Could you check a few things on this model? Use its own coordinates, in mm. Round coordinates to 2 decimals unless told otherwise and drop trailing zeros. Write each loop counter-clockwise with the first axis right and the second up, starting at its lowest first coordinate (ties: lowest second). Pieces come first, ordered by that corner, then holes. Notation, with made-up numbers: (49, 52) - (73, 52) arc R7 cw to (73, 63) - close; hole circle Ø7 at (-10, 29). An arc over 180 degrees is marked (long way). Put each result on its own line as item: value.
from build123d import *

# Parameters (mm, degrees)
SKETCH1_W                   = 50.8
SKETCH1_H                   = 88.500000038
SKETCH1_R                   = 14.2621
BOSS_EXTRUDE1_DEPTH         = 3.175
FILLET1_R                   = 5.08
F_1_4_0_25_DIAMETER_HOLE2_D = 6.35


with BuildPart() as part:
    # Sketch1 → Boss-Extrude1 (new, symmetric)
    with BuildSketch(Plane(origin=(0, 0, 0), x_dir=(0, 0, -1), z_dir=(1, 0, 0))):
        Rectangle(SKETCH1_W, SKETCH1_H)
        with Locations((0, -12.500000019)):
            Circle(SKETCH1_R, mode=Mode.SUBTRACT)
    extrude(amount=BOSS_EXTRUDE1_DEPTH, both=True)

    # Fillet1
    fillet1_edges = [part.edges().sort_by_distance(p)[0] for p in [
        (0, -44.250000019, -25.4),
        (0, -44.250000019, 25.4),
        (0, 44.250000019, 25.4),
        (0, 44.250000019, -25.4),
    ]]
    fillet(fillet1_edges, radius=FILLET1_R)

    # 1/4 (0.25) Diameter Hole2 (through all)
    with Locations(Plane(origin=(3.175, -37.900000019, 19.05), x_dir=(0, 0, 1), z_dir=(1, 0, 0))):
        with Locations((0, 0), (-38.1, 0), (0, -69.650000038), (-38.1, -69.650000038)):
            Hole(F_1_4_0_25_DIAMETER_HOLE2_D / 2)


solid = part.part
(1) Imagine slicing it at C-C, the plane x = 1.25. List the corners of the cut face in (y, z) for me (3 decimals).
Values found:
outline: (-44.25, -20.32) arc R5.08 ccw to (-39.17, -25.4) - (39.17, -25.4) arc R5.08 ccw to (44.25, -20.32) - (44.25, 20.32) arc R5.08 ccw to (39.17, 25.4) - (-39.17, 25.4) arc R5.08 ccw to (-44.25, 20.32) - close; hole circle Ø6.35 at (-37.9, -19.05); hole circle Ø6.35 at (-37.9, 19.05); hole circle Ø28.524 at (-12.5, 0); hole circle Ø6.35 at (31.75, -19.05); hole circle Ø6.35 at (31.75, 19.05)
(2) Please list where these lines run through material, in increasing order: probe 1 along Y at (x, z) = (0, 19.05) (3 decimals); probe 2 along Y at (x, z) = (1.5, 20.5); probe 3 along Z at (x, y) = (-0.25, -37.9) (3 decimals). Write a range as from..to.
Values found:
probe 1: y = -44.25..-41.075, -34.725..28.575, 34.925..44.25
probe 2: y = -44.25..-40.72, -35.08..28.93, 34.57..44.25
probe 3: z = -25.4..-22.225, -15.875..15.875, 22.225..25.4
(3) Imagine slicing it at B-B, the plane z = 19.05. List the corners of the cut face in (x, y) for me (3 decimals).
Values found:
outline: (-3.175, -44.25) - (3.175, -44.25) - (3.175, -41.075) - (-3.175, -41.075) - close; (-3.175, -34.725) - (3.175, -34.725) - (3.175, 28.575) - (-3.175, 28.575) - close; (-3.175, 34.925) - (3.175, 34.925) - (3.175, 44.25) - (-3.175, 44.25) - close
(4) Imagine slicing it at D-D, the plane z = 0. List the corners of the cut face in (x, y) for me (3 decimals).
Values found:
outline: (-3.175, -44.25) - (3.175, -44.25) - (3.175, -26.762) - (-3.175, -26.762) - close; (-3.175, 1.762) - (3.175, 1.762) - (3.175, 44.25) - (-3.175, 44.25) - close
(5) I'm going to push a flat-ended pin straight in: pin 1 (8.5 mm diameter, centred on y = 31.75, z = -19.05, fed in from +X) (3 decimals). Where does the tip first touch, or does it pass through?
Values found:
pin 1: stops at x = 3.175
(6) If we mould it in two halves opening along Y, with no side actions, what happens to faces 1 (the face through (0, -1, -25.4)), 2 (the face through (-0.04, 28.6, -18.64)), 3 (the face through (-0.044, 42.722, -23.951))? For each: pulls with the +Y half, pulls with the -Y half, needs draft (parallel to the pull), parting line crosses it, or undercut.
Values found:
face 1: needs draft
face 2: undercut
face 3: pulls with the +Y half
(7) Imagine slicing it at A-A, the plane y = 31.75. List the corners of the cut face in (x, z) for me (3 decimals).
Values found:
outline: (-3.175, -25.4) - (3.175, -25.4) - (3.175, -22.225) - (-3.175, -22.225) - close; (-3.175, -15.875) - (3.175, -15.875) - (3.175, 15.875) - (-3.175, 15.875) - close; (-3.175, 22.225) - (3.175, 22.225) - (3.175, 25.4) - (-3.175, 25.4) - close
